```python
from build123d import *

# Parameters (mm, degrees)
SKETCH1_W           = 40
SKETCH1_H           = 50
BOSS_EXTRUDE1_DEPTH = 4
CUT_EXTRUDE2_DEPTH  = 33.26453161
SKETCH4_R           = 2.15
CUT_EXTRUDE3_DEPTH  = 33.26453161
SKETCH5_R           = 2.15
CUT_EXTRUDE4_DEPTH  = 33.26453161
SKETCH8_R           = 2.15
CUT_EXTRUDE5_DEPTH  = 33.26453161


with BuildPart() as part:
    # Sketch1 → Boss-Extrude1 (new body)
    with BuildSketch(Plane.XY):
        Rectangle(SKETCH1_W, SKETCH1_H)
    extrude(amount=BOSS_EXTRUDE1_DEPTH)

    # Sketch3 → Cut-Extrude2 (cut, through all)
    with BuildSketch(Plane.XY.offset(4)):
        Polygon((2.68, 25), (20, -5), (20, 25), align=None)
    extrude(amount=-CUT_EXTRUDE2_DEPTH, mode=Mode.SUBTRACT)

    # Sketch4 → Cut-Extrude3 (cut, through all)
    with BuildSketch(Plane.XY.offset(4)):
        with Locations((2.500165004, 7.990476321)):
            Circle(SKETCH4_R)
    extrude(amount=-CUT_EXTRUDE3_DEPTH, mode=Mode.SUBTRACT)

    # Sketch5 → Cut-Extrude4 (cut, through all)
    with BuildSketch(Plane.XY.offset(4)):
        with Locations((-10, -15)):
            Circle(SKETCH5_R)
    extrude(amount=-CUT_EXTRUDE4_DEPTH, mode=Mode.SUBTRACT)

    # Sketch8 → Cut-Extrude5 (cut, through all)
    with BuildSketch(Plane.XY.offset(4)):
        with Locations((10, -15)):
            Circle(SKETCH8_R)
    extrude(amount=-CUT_EXTRUDE5_DEPTH, mode=Mode.SUBTRACT)


solid = part.part
```
Input: part model. Units: mm. Frame: model coordinates. Coordinates: 2 decimals unless noted, no trailing zeros. Order: outer loops, then holes, each group sorted by start corner. A loop starts at its lowest first (then second) coordinate and runs counter-clockwise, first axis right, second up. Notation, with made-up numbers: (-14.5, 39) - (-1.5, 39) arc R10 cw to (-1.5, 50) - close; hole circle Ø1 at (10, 7.25). An arc over 180 degrees is marked (long way). Put each result on its own line as item: value.
1. Contact query for flat-ended pins moving along their axis: pin 1 Ø4 at (x, y) = (2.5, 2) entering from -Z; pin 2 Ø1.5 at (y, z) = (18, 2.5) entering from +X. Output: stop coordinate, or through.
Report:
pin 1: stops at z = 0
pin 2: stops at x = 7.15
2. Cut plane D-D on x = 10. Return the cut outline in (y, z), then the cut area to 3 significant figures.
Report:
outline: (-25, 0) - (-17.15, 0) - (-17.15, 4) - (-25, 4) - close; (-12.85, 0) - (12.32, 0) - (12.32, 4) - (-12.85, 4) - close
area: 132 mm2
3. Cut plane C-C on z = 1.9. Return the cut outline in (x, y).
Report:
outline: (-20, -25) - (20, -25) - (20, -5) - (2.68, 25) - (-20, 25) - close; hole circle Ø4.3 at (-10, -15); hole circle Ø4.3 at (2.5, 7.99); hole circle Ø4.3 at (10, -15)
4. Cut plane A-A on x = -10. Return the cut outline in (y, z).
Report:
outline: (-25, 0) - (-17.15, 0) - (-17.15, 4) - (-25, 4) - close; (-12.85, 0) - (25, 0) - (25, 4) - (-12.85, 4) - close
5. Cut plane B-B on y = -15. Return the cut outline in (x, z), then the cut area to 3 significant figures.
Report:
outline: (-20, 0) - (-12.15, 0) - (-12.15, 4) - (-20, 4) - close; (-7.85, 0) - (7.85, 0) - (7.85, 4) - (-7.85, 4) - close; (12.15, 0) - (20, 0) - (20, 4) - (12.15, 4) - close
area: 126 mm2
6. Line query: line 1 along Y through (x, z) = (-10, 1.85); line 2 along X through (y, z) = (7, 0.3); line 3 along X through (y, z) = (-13.5, 0.6). Output: solid intervals per line, ascending.
Report:
line 1: y = -25 to -17.15, -12.85 to 25
line 2: x = -20 to 0.59, 4.41 to 13.07
line 3: x = -20 to -11.54, -8.46 to 8.46, 11.54 to 20
